Autodesk Inventor part; units mm, degrees
ref_plane "YZ Plane" through (0, 0, 0) normal (1, 0, 0) x (0, 1, 0)
ref_plane "XZ Plane" through (0, 0, 0) normal (0, 1, 0) x (-1, 0, 0)
ref_plane "XY Plane" through (0, 0, 0) normal (0, 0, 1) x (1, 0, 0)
sketch "Sketch1" plane through (0, 0, 0) normal (0, 1, 0) x (-1, 0, 0)
  line L0 (0.25, 0.25) -> (-0.25, 0.25)
  line L1 (-0.25, 0.25) -> (-0.25, -0.25)
  line L2 (-0.25, -0.25) -> (0.25, -0.25)
  line L3 (0.25, -0.25) -> (0.25, 0.25)
  line L4 (0.25, 0.25) -> (-0.25, -0.25) construction
  line L5 (-0.25, 0.25) -> (0.25, -0.25) construction
  point P0 (0, 0)
  dimension "d0" = 0.5
  dimension "d1" = 0.5
extrude "Extrusion1" add sketch "Sketch1" along normal blind 15.45
sketch "Sketch2" plane through (-0.25, 0, 0.25) normal (0, 0, 1) x (1, 0, 0)
  line L0 (0, 0) -> (0, 15.45)
  line L1 (0.5, 0) -> (0.5, 15.45)
  line L2 (0, 15.45) -> (0.5, 15.45)
  line L3 (0.5, 15.45) -> (0.5, 14.95)
  line L4 (0.5, 14.95) -> (0, 14.95)
  line L5 (0, 14.95) -> (0, 15.45)
  point P0 (0.25, 0)
  point P1 (0, 14.95)
  dimension "d4" = 0.5
extrude "Extrusion2" add sketch "Sketch2" along normal blind 0.3
properties part number "jst-ph-5p_wire"
Geometry: final body of the model. Coordinates: model frame, mm. Give positions to 0.01 mm unless a question says otherwise; leave off trailing zeros. Write each loop counter-clockwise with the first axis right and the second up, starting at its lowest first coordinate (ties: lowest second). Pieces come first, ordered by that corner, then holes. Notation, with made-up numbers: M -28,66.5 L -5,66.5 A18 cw -5,83.5 Z; hole C 4.5,55.25 d5. An arc over 180 degrees is marked long. Answer in a Markdown table with one row per item. Add a question column.
(1) Ray query, line 1 (Z direction, x = -0.2, y = 10.25); line 2 (Y direction, x = -0.05, z = 0.3). Return the intervals inside material, ascending.
(2) Section A-A on x = -0.1. Return loops of the section in (y, z).
(3) Section C-C on z = 0.4. Return loops of the section in (x, y), and give its area (3 significant figures).
(4) Section B-B on y = 9.5. Return loops of the section in (x, z).
Result set:
| question | item | result |
|---|---|---|
| 1 | line 1 | z = -0.25 to 0.25 |
| 1 | line 2 | y = 14.95 to 15.45 |
| 2 | outline | M 0,-0.25 L 15.45,-0.25 L 15.45,0.55 L 14.95,0.55 L 14.95,0.25 L 0,0.25 Z |
| 3 | outline | M -0.25,14.95 L 0.25,14.95 L 0.25,15.45 L -0.25,15.45 Z |
| 3 | area | 0.250 mm^2 |
| 4 | outline | M -0.25,-0.25 L 0.25,-0.25 L 0.25,0.25 L -0.25,0.25 Z |
